Design review of the part built by this model. Coordinates are the model's own, in mm. A direction names the side the tool comes from. Give positions to 0.01 mm unless a question says otherwise; leave off trailing zeros. Order: outer loops, then holes, each group sorted by start corner. A loop starts at its lowest first (then second) coordinate and runs counter-clockwise, first axis right, second up. Notation, with made-up numbers: (-28.5, -26) - (8.5, -26) arc R29 cw to (8.5, 0) - close; hole circle Ø1 at (55.25, 9). An arc over 180 degrees is marked (long way). Write each question's results on one line, items separated by ' | '. Start each with the question number.
```python
from build123d import *

# Parameters (mm, degrees)
SKIZZE1_W                       = 50
SKIZZE1_H                       = 50
SKIZZE1_R                       = 1.25
AUFSATZ_LINEAR_AUSTRAGEN1_DEPTH = 1.7
VERRUNDUNG1_R                   = 2
SKIZZE2_W                       = 14
SKIZZE2_H                       = 14
SKIZZE2_W_2                     = 7
SKIZZE2_H_2                     = 7
SKIZZE2_W_3                     = 5
SKIZZE2_H_3                     = 6
AUFSATZ_LINEAR_AUSTRAGEN2_DEPTH = 2
SKIZZE3_W                       = 4
SKIZZE3_H                       = 8
AUFSATZ_LINEAR_AUSTRAGEN3_DEPTH = 5
SKIZZE5_W                       = 5.5
SKIZZE5_H                       = 3
AUFSATZ_LINEAR_AUSTRAGEN5_DEPTH = 4.5
SKIZZE6_W                       = 5.5
SKIZZE6_H                       = 8
AUFSATZ_LINEAR_AUSTRAGEN6_DEPTH = 3.6


with BuildPart() as part:
    # Skizze1 → Aufsatz-Linear austragen1 (new body)
    with BuildSketch(Plane.XY):
        Rectangle(SKIZZE1_W, SKIZZE1_H)
        with Locations((-23, 23)):
            Circle(SKIZZE1_R, mode=Mode.SUBTRACT)
        with Locations((23, 23)):
            Circle(SKIZZE1_R, mode=Mode.SUBTRACT)
        with Locations((23, -23)):
            Circle(SKIZZE1_R, mode=Mode.SUBTRACT)
        with Locations((-23, -23)):
            Circle(SKIZZE1_R, mode=Mode.SUBTRACT)
    extrude(amount=AUFSATZ_LINEAR_AUSTRAGEN1_DEPTH)

    # Verrundung1
    verrundung1_edges = [part.edges().sort_by_distance(p)[0] for p in [
        (25, 25, 0.85),
        (25, -25, 0.85),
        (-25, -25, 0.85),
        (-25, 25, 0.85),
    ]]
    fillet(verrundung1_edges, radius=VERRUNDUNG1_R)

    # Skizze2 → Aufsatz-Linear austragen2 (add)
    with BuildSketch(Plane.XY.offset(1.7)):
        with Locations((11.5, 0)):
            Rectangle(SKIZZE2_W, SKIZZE2_H)
        with Locations((-5.5, 6)):
            Rectangle(SKIZZE2_W_2, SKIZZE2_H_2)
        with Locations((-5.5, -6)):
            Rectangle(SKIZZE2_W_2, SKIZZE2_H_2)
        with Locations((-10.7, 18)):
            Rectangle(SKIZZE2_W_3, SKIZZE2_H_3)
        with Locations((-16.5, 18)):
            Rectangle(SKIZZE2_W_3, SKIZZE2_H_3)
        with Locations((-4.9, 18)):
            Rectangle(SKIZZE2_W_3, SKIZZE2_H_3)
        with Locations((0.9, 18)):
            Rectangle(SKIZZE2_W_3, SKIZZE2_H_3)
        with Locations((6.7, 18)):
            Rectangle(SKIZZE2_W_3, SKIZZE2_H_3)
        with Locations((12.5, 18)):
            Rectangle(SKIZZE2_W_3, SKIZZE2_H_3)
        with Locations((12.5, -18)):
            Rectangle(SKIZZE2_W_3, SKIZZE2_H_3)
        with Locations((6.7, -18)):
            Rectangle(SKIZZE2_W_3, SKIZZE2_H_3)
        with Locations((0.9, -18)):
            Rectangle(SKIZZE2_W_3, SKIZZE2_H_3)
        with Locations((-4.9, -18)):
            Rectangle(SKIZZE2_W_3, SKIZZE2_H_3)
        with Locations((-10.7, -18)):
            Rectangle(SKIZZE2_W_3, SKIZZE2_H_3)
        with Locations((-16.5, -18)):
            Rectangle(SKIZZE2_W_3, SKIZZE2_H_3)
    extrude(amount=AUFSATZ_LINEAR_AUSTRAGEN2_DEPTH)

    # Skizze3 → Aufsatz-Linear austragen3 (add)
    with BuildSketch(Plane.XY.offset(1.7)):
        with Locations((-22.2, -4.5)):
            Rectangle(SKIZZE3_W, SKIZZE3_H)
        with Locations((-22.2, 4.5)):
            Rectangle(SKIZZE3_W, SKIZZE3_H)
    extrude(amount=AUFSATZ_LINEAR_AUSTRAGEN3_DEPTH)

    # Skizze5 → Aufsatz-Linear austragen5 (add)
    with BuildSketch(Plane.XY.offset(1.7)):
        with Locations((17.817192877, -22.933750346)):
            Rectangle(SKIZZE5_W, SKIZZE5_H)
    extrude(amount=AUFSATZ_LINEAR_AUSTRAGEN5_DEPTH)

    # Skizze6 → Aufsatz-Linear austragen6 (add)
    with BuildSketch(Plane(origin=(0, 0, 0), x_dir=(-1, 0, 0), z_dir=(0, 0, -1))):
        with Locations((25.45, 15.25)):
            Rectangle(SKIZZE6_W, SKIZZE6_H)
        with Locations((25.45, -15.25)):
            Rectangle(SKIZZE6_W, SKIZZE6_H)
        with Locations((-25.45, -9.5)):
            Rectangle(SKIZZE6_W, SKIZZE6_H)
    extrude(amount=AUFSATZ_LINEAR_AUSTRAGEN6_DEPTH)


solid = part.part
```
Q1. Add section A-A (z = 5.25). Give the boundary of the cut face in (x, y).
Q2. Machinability: for faces 5 (the flat face through (3.4, -18, 3)), 6 (the flat face through (-7.4, 18, 3)), 7 (the flat face through (7, 21, 3)), 8 (the flat face through (-22, 0.5, 4)), which of the approach directions +Z, -Z, +X, -X, +Y, -Y give a long, thin tool a straight path to every point of the face, cutting with its end or side? Answer none if there is none.
Q3. Add section B-B (x = 2.5). Give the boundary of the cut face in (y, z).
Q4. Draft analysis for pull direction Y (two halves, no side actions). For faces 1 (the flat face through (11, -7, 3)), 2 (the flat face through (-17, 15, 3)), 3 (the flat face through (-17, -21, 3)), 4 (the cylindrical face through (24.4, 24.43, 0.86)), state which applies: pulls with the +Y half, pulls with the -Y half, needs draft (parallel to the pull), parting line crosses it, or undercut.
Q5. Insertion check: pin 1 Ø3 at (x, y) = (-15.5, -18.5) entering from +Z; pin 2 Ø0.6 at (y, z) = (-19, 3) entering from +X; pin 3 Ø2 at (y, z) = (-7, 2.5) entering from -X. Each pin has a flat end and moves straight along its axis. Give the tip position at first contact, or say it passes through.
Q6. Add section D-D (z = 2.5). Give the number of separate pieces and of enclosed holes in the cut face, plus the area to 4 significant figures.
Q7. For line 1 (Y direction, x = 23, z = 0.6); line 2 (Y direction, x = -16.5, z = 3); line 3 (X direction, y = 7, z = 0.5), list the stretches that pass through material, from the lowest coordinate up. Write a range as [from, to].
Q8. Add section C-C (z = -2). Give the boundary of the cut face in (x, y).
Verdict:
1) outline: (-24.2, -8.5) - (-20.2, -8.5) - (-20.2, -0.5) - (-24.2, -0.5) - close; (-24.2, 0.5) - (-20.2, 0.5) - (-20.2, 8.5) - (-24.2, 8.5) - close; (15.07, -24.43) - (20.57, -24.43) - (20.57, -21.43) - (15.07, -21.43) - close
2) face 5: +Z, +Y, -Y | face 6: +Z, +Y | face 7: +Z, +X, -X, +Y | face 8: +Z, -X
3) outline: (-25, 0) - (25, 0) - (25, 1.7) - (21, 1.7) - (21, 3.7) - (15, 3.7) - (15, 1.7) - (-15, 1.7) - (-15, 3.7) - (-21, 3.7) - (-21, 1.7) - (-25, 1.7) - close
4) face 1: undercut | face 2: undercut | face 3: pulls with the -Y half | face 4: pulls with the +Y half
5) pin 1: stops at z = 3.7 | pin 2: stops at x = 15 | pin 3: stops at x = -25
6) separate pieces: 18 | enclosed holes: 0 | area: 734.5 mm2
7) line 1: y = [-25, -24.25], [-21.75, 21.75], [24.25, 25] | line 2: y = [-21, -15], [15, 21] | line 3: x = [-25, 25]
8) outline: (-28.2, -19.25) - (-22.7, -19.25) - (-22.7, -11.25) - (-28.2, -11.25) - close; (-28.2, 11.25) - (-22.7, 11.25) - (-22.7, 19.25) - (-28.2, 19.25) - close; (22.7, -13.5) - (28.2, -13.5) - (28.2, -5.5) - (22.7, -5.5) - close
